Autodesk Inventor part; units mm, degrees
ref_plane "YZ Plane" through (0, 0, 0) normal (1, 0, 0) x (0, 1, 0)
ref_plane "XZ Plane" through (0, 0, 0) normal (0, 1, 0) x (-1, 0, 0)
ref_plane "XY Plane" through (0, 0, 0) normal (0, 0, 1) x (1, 0, 0)
sketch "Skizze1" plane through (0, 0, 0) normal (0, 0, 1) x (1, 0, 0)
  line L0 (0, 0) -> (0, 22.5)
  line L1 (0, 22.5) -> (5, 22.5)
  line L2 (5, 22.5) -> (5, 12)
  line L3 (5, 12) -> (7.9, 12)
  line L4 (7.9, 12) -> (7.9, 9.5)
  line L5 (7.9, 9.5) -> (3, 9.5)
  line L6 (3, 9.5) -> (3, 0)
  line L7 (3, 0) -> (0, 0)
  line L8 (5, 17.25) -> (0, 17.25) construction
  line L9 (0, 18.75) -> (5, 18.75) construction
  line L10 (0, 15.75) -> (5, 15.75) construction
  line L11 (9, 12) -> (9, 0) construction
  line L12 (5, 12) -> (5, 0) construction
  dimension "d0" = 19
  dimension "d3" = 5
  dimension "d5" = 3
  dimension "d6" = 1.5
  dimension "d7" = 3.75
  dimension "d17" = 2.5
  dimension "d18" = 24
  dimension "d31" = 1.1
  dimension "d32" = 4
  dimension "d33" = 2
  dimension "d34" = 3
  dimension "DrivenPart_Flansch_TotalThickness" = 9
  dimension "d41" = 45
  dimension "FixationHole_Dia" = 34.5
revolve "Umdrehung1" add sketch "Skizze1" angle 360 about axis through (3, 0, 0) along (-1, 0, 0)
sketch "Skizze4" plane through (5, 0, 0) normal (1, 0, 0) x (0, -1, 0)
  line L0 (-14.0557, 10) -> (14.0557, 10) construction
  line L1 (14.0557, 10) -> (14.0557, -10) construction
  line L2 (14.0557, -10) -> (-14.0557, -10) construction
  line L3 (-14.0557, -10) -> (-14.0557, 10) construction
  circle A0 centre (0, 0) radius 12 construction
  line L4 (-14.0557, 10) -> (14.0557, -10) construction
  line L5 (14.0557, 10) -> (-14.0557, -10) construction
  circle A1 centre (0, 0) radius 17.25 construction
  arc A2 (-22.5, 0) -> (-22.5, 0) centre (0, 0) ccw construction
  circle A3 centre (0, 0) radius 22.5 construction
  dimension "d40" = 45
  dimension "d43" = 34.5
  dimension "d38" = 20
  dimension "d39" = 24
hole "Bohrung2" at (5, 14.0557, 10) at (5, 14.0557, -10) at (5, -14.0557, 10) at (5, -14.0557, -10) direction (-1, 0, 0) diameter 4.5 end through all countersink diameter 10 countersink angle 90
sketch "Skizze5" plane through (5, 0, 0) normal (1, 0, 0) x (0, 0, -1)
  circle A0 centre (0, 0) radius 22.5
  circle A1 centre (0, 0) radius 22.5
  line L0 (-20, -10.3078) -> (-20, 10.3078)
  line L1 (20, -10.3078) -> (20, 10.3078)
  point P0 (0, 0)
  dimension "d51" = 40
extrude "Extrusion2" cut sketch "Skizze5" against normal through all contours A0 L1 | L0 A0
sketch "Skizze6" plane through (7.9, 0, 0) normal (1, 0, 0) x (0, 0, -1)
  line L0 (-2.5, 18.7367) -> (2.5, 18.7367)
  line L1 (2.5, 18.7367) -> (2.5, 11.7367)
  line L2 (2.5, 11.7367) -> (-2.5, 11.7367)
  line L3 (-2.5, 11.7367) -> (-2.5, 18.7367)
  line L4 (0, 0) -> (0, 18.7367) construction
  circle A0 centre (0, 0) radius 12
  dimension "d54" = 5
  dimension "d55" = 7
extrude "Extrusion3" add sketch "Skizze6" against normal up to surface (2.9 mm away) contours L0 L1 A0 L3
sketch "Skizze7" plane through (7.9, 11.7367, 2.5) normal (0, 0, 1) x (1, 0, 0)
  line L0 (0, 7) -> (-2.9, 7)
  line L1 (0, 0) -> (-2.9, 0)
  line L2 (-2.9, 7) -> (0, 0)
  line L3 (0, 7) -> (0, 0)
  point P0 (-7.9, -11.7367)
extrude "Extrusion4" cut sketch "Skizze7" against normal through all
pattern_circular "Runde Anordnung1" count 4 over 360 about axis through (5.45, 0, 0) along (1, 0, 0) of "Extrusion3", "Extrusion4"
equation "\"d43\" = FixationHole_Dia"
equation "\"d6\" = 0.5 * d5"
properties part number "ParallelMecha_DrivenLink_ShaftFixation" material "Aluminium 6061"
The listing builds one solid part. Answer for the finished solid, in the listing's coordinates (mm). A direction names the side the tool comes from. Give positions to 0.01 mm unless a question says otherwise; leave off trailing zeros. Write each loop counter-clockwise with the first axis right and the second up, starting at its lowest first coordinate (ties: lowest second). Pieces come first, ordered by that corner, then holes.
Item 1: Section A-A, the plane z = -10 is taken. Write down the section's boundary in (x, y).
Item 2: Section B-B, the plane z = 0 is taken. Write down the section's boundary in (x, y).
Item 3: Section D-D, the plane x = 1.25 is taken. Write down the section's boundary in (y, z), plus the area to 3 significant figures.
Item 4: Determine the mould class of faces 1 (the cylindrical face through (6.47, -8.42, 8.55)), 2 (the cylindrical face through (6.47, 8.42, -8.55)), 3 (the flat face through (6, -14, 2.5)), 4 (the conical face through (2.42, -15.53, -8.08)) for opening direction Y: released by +Y, released by -Y, zero draft, split by the parting line, or undercut.
Item 5: Find the intervals of material crossed by line 1 along Y through (x, z) = (4.15, 0); line 2 along Y through (x, z) = (1.4, 10); line 3 along Y through (x, z) = (4.75, 7), in increasing order.
Item 6: Flat-ended cylindrical pins translate along their axes: P1, Ø2.5, axis at x = 6.5, y = -17, coming from the +Z side; P2, Ø9.5, axis at y = -1.5, z = 4, coming from the +X side; P3, Ø1, axis at x = 4.5, z = -14, coming from the -Y side; P4, Ø4, axis at y = 14.06, z = -10, coming from the -X side (3 decimals). Find the tip coordinate at first contact, or state that the pin passes through.
Item 7: Section C-C, the plane y = 0 is taken. Write down the section's boundary in (x, z), plus the area to 3 significant figures.
Item 8: Which of the six approach directions +Z, -Z, +X, -X, +Y, -Y give full straight-line access (tool end or side, diameter ignored) to faces 5 (the cylindrical face through (5.42, 4.38, 8.43)), 6 (the cylindrical face through (6.47, -8.55, -8.42)), 7 (the flat face through (6, 14, 2.5))?
Completed:
1. outline: (0, -20.16) - (5, -20.16) - (5, -19.06) - (2.25, -16.31) - (0, -16.31) - close; (0, -11.81) - (2.25, -11.81) - (5, -9.06) - (5, -6.63) - (7.9, -6.63) - (7.9, 6.63) - (5, 6.63) - (5, 9.06) - (2.25, 11.81) - (0, 11.81) - close; (0, 16.31) - (2.25, 16.31) - (5, 19.06) - (5, 20.16) - (0, 20.16) - close
2. outline: (0, -22.5) - (5, -22.5) - (5, -18.74) - (7.9, -11.74) - (7.9, -9.5) - (3, -9.5) - (3, 9.5) - (7.9, 9.5) - (7.9, 11.74) - (5, 18.74) - (5, 22.5) - (0, 22.5) - close
3. outline: (-10.31, -20) - (10.31, -20) arc R22.5 ccw to (10.31, 20) - (-10.31, 20) arc R22.5 ccw to start; hole circle Ø4.5 at (-14.06, -10); hole circle Ø4.5 at (-14.06, 10); hole circle Ø4.5 at (14.06, -10); hole circle Ø4.5 at (14.06, 10)
3. area: 1,460 mm2
4. face 1: released by -Y
4. face 2: released by +Y
4. face 3: zero draft
4. face 4: undercut
5. line 1: y = -22.5 to -9.5, 9.5 to 22.5
5. line 2: y = -20.16 to -16.31, -11.81 to 11.81, 16.31 to 20.16
5. line 3: y = -21.38 to -17.74, -10.37 to -6.42, 6.42 to 10.37, 17.74 to 21.38
6. P1: stops at z = 2.5
6. P2: stops at x = 3
6. P3: stops at y = -18
6. P4: passes through
7. outline: (0, -20) - (5, -20) - (5, -18.74) - (7.9, -11.74) - (7.9, -9.5) - (3, -9.5) - (3, 9.5) - (7.9, 9.5) - (7.9, 11.74) - (5, 18.74) - (5, 20) - (0, 20) - close
7. area: 195 mm2
8. face 5: +X
8. face 6: -Z, +X, -Y
8. face 7: +Z, +X, +Y
